Could you check a few things on this model? Use its own coordinates, in mm. Give positions to 0.01 mm unless a question says otherwise; leave off trailing zeros. Write each loop counter-clockwise with the first axis right and the second up, starting at its lowest first coordinate (ties: lowest second). Pieces come first, ordered by that corner, then holes. Notation, with made-up numbers: (20, 45.25) - (44, 45.25) arc R36 ccw to (44, 83.25) - close; hole circle Ø5 at (40.25, -28.75). An arc over 180 degrees is marked (long way). Answer in a Markdown table with one row per item.
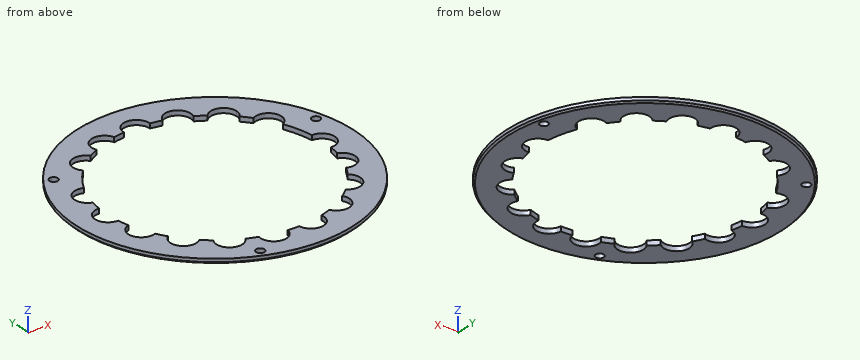
from build123d import *

# Parameters (mm, degrees)
F0_R     = 17.4791666667
F0_R_2   = 0.525
F1_DEPTH = 0.6
F2_SIZE  = 0.2
F3_SCALE = 3


with BuildPart() as f1:
    # F0 (on Top) → F1 (new body)
    with BuildSketch(Plane.XY):
        Circle(F0_R)
        with Locations((-5.6091303505, -15.4109589809)):
            Circle(F0_R_2, mode=Mode.SUBTRACT)
        with BuildLine():
            ThreePointArc((12.4211490883, 5.28819963), (13.0398483265, 3.494618094), (13.400990099, 1.6320123671))
            ThreePointArc((13.400990099, 1.6320123671), (14.5981493335, 1.1779324057), (15.1, 0))
            ThreePointArc((15.1, 0), (14.5981493335, -1.1779324057), (13.400990099, -1.6320123671))
            ThreePointArc((13.400990099, -1.6320123671), (13.2945098091, -2.3464886393), (13.1499649563, -3.0542464943))
            ThreePointArc((13.1499649563, -3.0542464943), (13.9724997299, -3.6467176264), (14.2870667184, -4.6103737402))
            ThreePointArc((14.2870667184, -4.6103737402), (13.5629249977, -5.9672629728), (12.0325993029, -6.1209928947))
            ThreePointArc((12.0325993029, -6.1209928947), (11.6880692654, -6.7556670173), (11.3100935731, -7.3710096574))
            ThreePointArc((11.3100935731, -7.3710096574), (11.7786571464, -7.9438467562), (11.9463186252, -8.6646683655))
            ThreePointArc((11.9463186252, -8.6646683655), (10.9714810033, -10.1593794332), (9.210611063, -9.8698857058))
            ThreePointArc((9.210611063, -9.8698857058), (8.6699484839, -10.3480429689), (8.1045033915, -10.7966209889))
            ThreePointArc((8.1045033915, -10.7966209889), (8.2948880144, -11.2170122777), (8.3600844859, -11.6738761091))
            ThreePointArc((8.3600844859, -11.6738761091), (7.1138213291, -13.2606824792), (5.2768749477, -12.4259643806))
            ThreePointArc((5.2768749477, -12.4259643806), (4.6057092155, -12.6900529007), (3.9213971545, -12.9179195057))
            ThreePointArc((3.9213971545, -12.9179195057), (3.9510070235, -13.0953907943), (3.9609170652, -13.2750421058))
            ThreePointArc((3.9609170652, -13.2750421058), (2.4309982831, -14.9050983037), (0.7073457896, -13.4814562245))
            ThreePointArc((0.7073457896, -13.4814562245), (-0.0130943041, -13.4999936496), (-0.7334970815, -13.4800586806))
            ThreePointArc((-0.7334970815, -13.4800586806), (-2.6390844274, -14.8832879588), (-3.9460263226, -12.9104173543))
            ThreePointArc((-3.9460263226, -12.9104173543), (-4.6288343322, -12.6816360429), (-5.2984716212, -12.4167708555))
            ThreePointArc((-5.2984716212, -12.4167708555), (-7.5709419973, -13.0876933984), (-8.1222459609, -10.783279675))
            ThreePointArc((-8.1222459609, -10.783279675), (-8.6853165754, -10.3351476034), (-9.2237075057, -9.8576477848))
            ThreePointArc((-9.2237075057, -9.8576477848), (-11.5911782598, -9.713769738), (-11.3188073747, -7.3576218723))
            ThreePointArc((-11.3188073747, -7.3576218723), (-11.6946164061, -6.744327032), (-12.0372272938, -6.1118867037))
            ThreePointArc((-12.0372272938, -6.1118867037), (-14.2150797243, -5.168494422), (-13.1517324298, -3.0466266746))
            ThreePointArc((-13.1517324298, -3.0466266746), (-13.2952994905, -2.3420101316), (-13.4011439404, -1.6307486284))
            ThreePointArc((-13.4011439404, -1.6307486284), (-15.1263287229, 0), (-13.4011439404, 1.6307486284))
            ThreePointArc((-13.4011439404, 1.6307486284), (-13.2952994905, 2.3420101316), (-13.1517324298, 3.0466266746))
            ThreePointArc((-13.1517324298, 3.0466266746), (-14.2150797243, 5.168494422), (-12.0372272938, 6.1118867037))
            ThreePointArc((-12.0372272938, 6.1118867037), (-11.0598636595, 7.7414091633), (-9.8633913446, 9.217565361))
            ThreePointArc((-9.8633913446, 9.217565361), (-9.7217308873, 11.5859077112), (-7.3647698988, 11.3141576946))
            ThreePointArc((-7.3647698988, 11.3141576946), (-6.75, 11.6913429511), (-6.1159630365, 12.0351566727))
            ThreePointArc((-6.1159630365, 12.0351566727), (-5.1728249601, 14.2122197728), (-3.0509500914, 13.1507301523))
            ThreePointArc((-3.0509500914, 13.1507301523), (-2.3442503985, 13.2949046657), (-1.6308593243, 13.4011304696))
            ThreePointArc((-1.6308593243, 13.4011304696), (-0.0449493128, 15.1237097603), (1.6333333333, 13.4909950464))
            ThreePointArc((1.6333333333, 13.4909950464), (1.6327147139, 13.4460457336), (1.6308593243, 13.4011304696))
            ThreePointArc((1.6308593243, 13.4011304696), (2.3442503985, 13.2949046657), (3.0509500914, 13.1507301523))
            ThreePointArc((3.0509500914, 13.1507301523), (4.8534435624, 14.2931039672), (6.2475253927, 12.6773884922))
            ThreePointArc((6.2475253927, 12.6773884922), (6.2142968019, 12.3496041257), (6.1159630365, 12.0351566727))
            ThreePointArc((6.1159630365, 12.0351566727), (6.75, 11.6913429511), (7.3647698988, 11.3141576946))
            ThreePointArc((7.3647698988, 11.3141576946), (9.1880272411, 11.8843253264), (10.3051777915, 10.3347017875))
            ThreePointArc((10.3051777915, 10.3347017875), (10.1907208563, 9.7340419295), (9.8633913446, 9.217565361))
            ThreePointArc((9.8633913446, 9.217565361), (10.3415999821, 8.6776327308), (10.790289764, 8.1129308397))
            ThreePointArc((10.790289764, 8.1129308397), (12.4609745427, 8.181944599), (13.3168777659, 6.7454975232))
            ThreePointArc((13.3168777659, 6.7454975232), (13.0750421955, 5.8902129195), (12.4211490883, 5.28819963))
        make_face(mode=Mode.SUBTRACT)
        with Locations((-13.4340935263, 9.4066535562)):
            Circle(F0_R_2, mode=Mode.SUBTRACT)
        with Locations((15.8411835511, 4.2446323397)):
            Circle(F0_R_2, mode=Mode.SUBTRACT)
    extrude(amount=F1_DEPTH)

    # F2
    f2_edges = [f1.edges().sort_by_distance(p)[0] for p in [
        (-17.479167, 0, 0),
    ]]
    chamfer(f2_edges, length=F2_SIZE)


with BuildPart() as f1_1:
    # F3: moved
    add(f1.part.scale(F3_SCALE))


solid = f1_1.part
1) Imagine slicing it at B-B (z = 1.15). State how many separate pieces and enclosed holes the cut face has, then the cut area to 3 significant figures.
Check values:
| item | result |
|---|---|
| separate pieces | 1 |
| enclosed holes | 4 |
| area | 2,810 mm2 |
2) Imagine slicing it at A-A (x = 0). List the corners of the cut face in (y, z) for me.
Check values:
| item | result |
|---|---|
| outline | (-52.44, 0.6) - (-51.84, 0) - (-40.5, 0) - (-40.5, 1.8) - (-52.44, 1.8) - close; (45.37, 0) - (51.84, 0) - (52.44, 0.6) - (52.44, 1.8) - (45.37, 1.8) - close |
3) If I drill on line 1 (X direction, y = 42, z = 1.7); line 2 (X direction, y = 23, z = 0.8); line 3 (Y direction, x = 31, z = 0.2), over which ranges is the centre line in solid material (lowest first)?
Check values:
| item | result |
|---|---|
| line 1 | x = -31.4 to -16.72, -10.97 to -4.66, 4.66 to 10.97, 16.72 to 31.4 |
| line 2 | x = -47.12 to -33.34, 39.1 to 47.12 |
| line 3 | y = -41.8 to -30.89, 26.06 to 41.8 |
4) Will these pins go through, and if not, where does the flat tip stop? P1, Ø2.5, axis at x = 47.52, y = 12.73, coming from the +Z side; P2, Ø1, axis at x = -36.5, z = 0.5, coming from the -Y side.
Check values:
| item | result |
|---|---|
| P1 | passes through |
| P2 | stops at y = -38.12 |
